from build123d import *

# Parameters (mm, degrees)
EXTRUDE_1_DEPTH     = 6
SKETCH_2_R          = 6.5
CUT_EXTRUDE_1_DEPTH = 56.865910894
CHAMFER_1_SIZE      = 1
CHAMFER_2_SIZE      = 2


with BuildPart() as part:
    # 草图1 → 凸台-拉伸1 (new, symmetric)
    with BuildSketch(Plane.XY):
        Polygon((0, -14), (0, 14), (5.373066959, 14), (5.373066959, 36), (23.373066959, 31.176914536), (41, 21), (41, -21), (23.373066959, -31.176914536), (5.373066959, -36), (5.373066959, -14), align=None)
    extrude(amount=EXTRUDE_1_DEPTH, both=True)

    # 草图2 → 切除-拉伸1 (cut, through all)
    with BuildSketch(Plane.XY.offset(6)):
        with Locations((23, 0)):
            Circle(SKETCH_2_R)
    extrude(amount=-CUT_EXTRUDE_1_DEPTH, mode=Mode.SUBTRACT)

    # 倒角1
    chamfer_1_edges = [part.edges().sort_by_distance(p)[0] for p in [
        (16.5, 0, -6),
        (16.5, 0, 6),
    ]]
    chamfer(chamfer_1_edges, length=CHAMFER_1_SIZE)

    # 倒角2
    chamfer_2_edges = [part.edges().sort_by_distance(p)[0] for p in [
        (14.373066959, -33.588457268, -6),
        (14.373066959, 33.588457268, -6),
        (32.186533479, 26.088457268, 6),
        (32.186533479, 26.088457268, -6),
        (32.186533479, -26.088457268, -6),
        (14.373066959, 33.588457268, 6),
        (14.373066959, -33.588457268, 6),
        (32.186533479, -26.088457268, 6),
    ]]
    chamfer(chamfer_2_edges, length=CHAMFER_2_SIZE)


solid = part.part
Design review of the part built by this model. Coordinates are the model's own, in mm. A direction names the side the tool comes from. Round coordinates to 2 decimals unless told otherwise and drop trailing zeros. Loops run counter-clockwise (first coordinate to the right, second up) from the corner with the lowest first, then second, coordinate; pieces in that order, holes last. Notation, with made-up numbers: (2.25, 79.5) - (27.25, 79.5) arc R21 cw to (27.25, 112.5) - close; hole circle Ø2 at (49, 64.5). An arc over 180 degrees is marked (long way). One line per item, written item: value. Start each with the question number.
1) Consider section C-C on x = 31.5. Give the boundary of the cut face in (y, z), then the cut area to 3 significant figures.
2) Insertion check: pin 1 Ø21 at (x, y) = (23, 0) entering from +Z; pin 2 Ø3 at (x, z) = (21, -3.5) entering from +Y; pin 3 Ø6 at (x, z) = (2, -0.5) entering from +Y; pin 4 Ø3.5 at (y, z) = (-22, 3) entering from -X. Each pin has a flat end and moves straight along its axis. Give the tip position at first contact, or say it passes through.
3) Consider section D-D on y = 27. Give the boundary of the cut face in (x, z), then the cut area to 3 significant figures.
4) Consider section A-A on y = 0. Give the boundary of the cut face in (x, z).
5) Consider section B-B on z = -0.75. Give the boundary of the cut face in (x, y), then the cut area to 3 significant figures.
6) To check wall thickness, follow L1, parallel to X at y = 15, z = 0.5; L2, parallel to Y at x = 23, z = -0.5; L3, parallel to X at y = -3.5, z = -2.25. State the ranges of each line that lie inside material, in increasing order. Write a range as from..to.
7) For faces 1 (the flat face through (3, -14, 0)), 2 (the flat face through (32.31, -26.017, 0.056)), 3 (the flat face through (3, 14, 0)), list the 3-axis set-ups (+Z, -Z, +X, -X, +Y, -Y) from which the entire face can be reached by the end or side of a thin tool; tool diameter is ignored.
Reported:
1. outline: (-26.48, -4) - (-24.18, -6) - (24.18, -6) - (26.48, -4) - (26.48, 4) - (24.18, 6) - (-24.18, 6) - (-26.48, 4) - close
1. area: 626 mm^2
2. pin 1: stops at z = 6
2. pin 2: stops at y = 32.21
2. pin 3: stops at y = 14
2. pin 4: stops at x = 5.37
3. outline: (5.37, -6) - (26.61, -6) - (30.61, -4) - (30.61, 4) - (26.61, 6) - (5.37, 6) - close
3. area: 295 mm^2
4. outline: (0, -6) - (15.5, -6) - (16.5, -5) - (16.5, 5) - (15.5, 6) - (0, 6) - close; (29.5, -5) - (30.5, -6) - (41, -6) - (41, 6) - (30.5, 6) - (29.5, 5) - close
5. outline: (0, -14) - (5.37, -14) - (5.37, -36) - (23.37, -31.18) - (41, -21) - (41, 21) - (23.37, 31.18) - (5.37, 36) - (5.37, 14) - (0, 14) - close; hole circle Ø13 at (23, 0)
5. area: 2,150 mm^2
6. L1: x = 5.37..41
6. L2: y = -31.28..-6.5, 6.5..31.28
6. L3: x = 0..17.52, 28.48..41
7. face 1: +Z, -Z, -X, -Y
7. face 2: +Z, -Z, +X, -Y
7. face 3: +Z, -Z, -X, +Y
